```python
from build123d import *

# Parameters (mm, degrees)
SKETCH1_W                   = 38
SKETCH1_H                   = 8
BOSS_EXTRUDE1_DEPTH         = 8
TAP_DRILL_FOR_M5X0_8_TAP1_D = 4.2
TAP_DRILL_FOR_M3X0_5_TAP1_D = 2.5
TAP_DRILL_FOR_M3X0_5_TAP2_D = 2.5


with BuildPart() as part:
    # Sketch1 → Boss-Extrude1 (new body)
    with BuildSketch(Plane.XY):
        with Locations((19, 4)):
            Rectangle(SKETCH1_W, SKETCH1_H)
    extrude(amount=BOSS_EXTRUDE1_DEPTH)

    # Tap Drill for M5x0.8 Tap1 (through all)
    with Locations(Plane(origin=(0, 8, 0), x_dir=(-1, 0, 0), z_dir=(0, 1, 0))):
        with Locations((-19, 4)):
            Hole(TAP_DRILL_FOR_M5X0_8_TAP1_D / 2)

    # Tap Drill for M3x0.5 Tap1 (through all)
    with Locations(Plane(origin=(0, 0, 0), x_dir=(-1, 0, 0), z_dir=(0, 0, -1))):
        with Locations((-35, 4), (-3, 4)):
            Hole(TAP_DRILL_FOR_M3X0_5_TAP1_D / 2)

    # Tap Drill for M3x0.5 Tap2 (through all)
    with Locations(Plane(origin=(0, 8, 0), x_dir=(-1, 0, 0), z_dir=(0, 1, 0))):
        with Locations((-11.5, 4), (-26.5, 4)):
            Hole(TAP_DRILL_FOR_M3X0_5_TAP2_D / 2)


solid = part.part
```
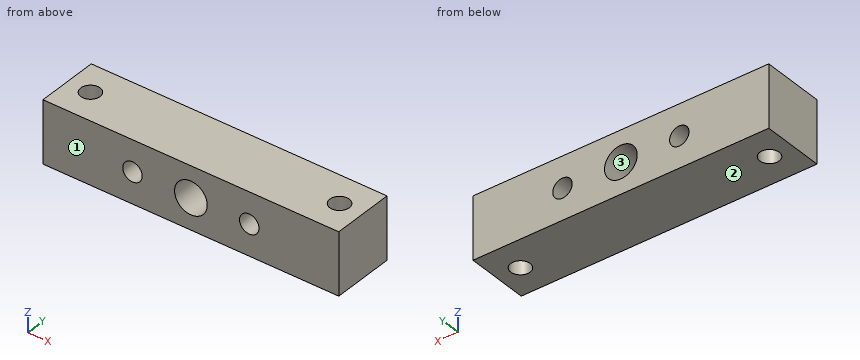
Build history of the part. All positions in model axes, mm. Face numbers are marked on the shaded views. Coordinates: 2 decimals unless noted, no trailing zeros. Write each loop counter-clockwise with the first axis right and the second up, starting at its lowest first coordinate (ties: lowest second). Pieces come first, ordered by that corner, then holes.
1. Drill centre lines: probe 1 along Y at (x, z) = (35, 2.5); probe 2 along X at (y, z) = (6.5, 3). Where is each one in solid material? Low to high.
Answer block:
probe 1: y = 0 to 2.75, 5.25 to 8
probe 2: x = 0 to 10.75, 12.25 to 17.15, 20.85 to 25.75, 27.25 to 38
2. Drop a flat-ended pin along its axis: pin 1 (2.5 mm diameter, centred on x = 19, z = 4, fed in from +Y). Give the stop position or say it passes through.
Answer block:
pin 1: passes through
3. Band-saw the part on D-D, the plane z = 1.5. Give the cut face in (x, y).
Answer block:
outline: (0, 0) - (38, 0) - (38, 8) - (0, 8) - close; hole circle Ø2.5 at (3, 4); hole circle Ø2.5 at (35, 4)
4. Pull direction Z, two halves, no side cores. Call the marked faces 1, 2 and 3: released by +Z, released by -Z, zero draft, split by the parting line, or undercut.
Answer block:
face 1: zero draft
face 2: released by -Z
face 3: undercut
5. Band-saw the part on A-A, the plane y = 4. Give the cut face in (x, z).
Answer block:
outline: (0, 0) - (1.75, 0) - (1.75, 8) - (0, 8) - close; (4.25, 0) - (33.75, 0) - (33.75, 8) - (4.25, 8) - close; (36.25, 0) - (38, 0) - (38, 8) - (36.25, 8) - close; hole circle Ø2.5 at (11.5, 4); hole circle Ø4.2 at (19, 4); hole circle Ø2.5 at (26.5, 4)
6. Band-saw the part on B-B, the plane x = 19. Give the cut face in (y, z).
Answer block:
outline: (0, 0) - (8, 0) - (8, 1.9) - (0, 1.9) - close; (0, 6.1) - (8, 6.1) - (8, 8) - (0, 8) - close
7. Band-saw the part on C-C, the plane y = 1. Give the cut face in (x, z), and give its area (3 significant figures).
Answer block:
outline: (0, 0) - (38, 0) - (38, 8) - (0, 8) - close; hole circle Ø2.5 at (11.5, 4); hole circle Ø4.2 at (19, 4); hole circle Ø2.5 at (26.5, 4)
area: 280 mm2
